Could you check a few things on this model? Use its own coordinates, in mm. A direction names the side the tool comes from. Give positions to 0.01 mm unless a question says otherwise; leave off trailing zeros. Order: outer loops, then holes, each group sorted by start corner. A loop starts at its lowest first (then second) coordinate and runs counter-clockwise, first axis right, second up. Notation, with made-up numbers: M -32.5,-37.75 L -20.5,-37.75 A15 ccw -20.5,-26.75 Z; hole C 78.5,-13.5 d11. An arc over 180 degrees is marked long. Use a Markdown table: item, result. Add a question column.
Item 1: I'm going to push flat-ended pins straight in: pin 1 Ø6 at (x, y) = (13, 15) entering from -Z; pin 2 Ø2.5 at (y, z) = (12.8, 17.5) entering from -X; pin 3 Ø2.5 at (x, z) = (12.5, 21) entering from +Y; pin 4 Ø1 at (y, z) = (4.5, 15) entering from +X. Where does each tip first touch, or does it pass through?
Item 2: For faces 4 (the face through (5, 13, 8)), 5 (the face through (14, 24, 21)), 6 (the face through (11.633, 15.095, 18.838)), which set-ups out of +Z, -Z, +X, -X, +Y, -Y let a thin tool reach every point of the face, with its end or its side?
Item 3: Suppose I cut it at B-B on y = 7.8. Write out the boundary of the cut face in (x, z).
Item 4: Suppose I cut it at A-A on x = 12.5. Write out the boundary of the cut face in (y, z).
Item 5: If we mould it in two halves opening along X, with no side actions, what happens to faces 1 (the face through (12, 19, 12.5)), 2 (the face through (12, 13, 25)), 3 (the face through (5, 3, 18))? For each: released by +X, released by -X, zero draft, split by the parting line, or undercut.
Item 6: If I drill on L1, parallel to Y at x = 16, z = 12.25; L2, parallel to Z at x = 15.5, y = 7.8; L3, parallel to X at y = 24.3, z = 21, over which ranges is the centre line in solid material (lowest first)? Write a range as from..to.
Item 7: Suppose I cut it at D-D on x = 4.5. Write out the boundary of the cut face in (y, z).
Item 8: Suppose I cut it at C-C on z = 11.5. Write out the boundary of the cut face in (x, y), plus the area to 4 significant figures.
from build123d import *

# Parameters (mm, degrees)
F0_W     = 25
F0_H     = 25
F1_DEPTH = 25
F2_R     = 4
F3_DEPTH = 12.5
F4_R     = 1.5
F5_DEPTH = 6
F6_R     = 1.5
F7_DEPTH = 5
F8_R     = 5.05
F9_DEPTH = 25.001


with BuildPart() as f1:
    # F0 (on Top) → F1 (new body)
    with BuildSketch(Plane.XY):
        with Locations((12.5, 12.5)):
            Rectangle(F0_W, F0_H)
    extrude(amount=F1_DEPTH)

    # F2 (on face) → F3 (cut)
    with BuildSketch(Plane.XY.offset(25)):
        with Locations((12.5, 19)):
            Circle(F2_R)
    extrude(amount=-F3_DEPTH, mode=Mode.SUBTRACT)

    # F4 (on face) → F5 (cut)
    with BuildSketch(Plane(origin=(0, 25, 0), x_dir=(-1, 0, 0), z_dir=(0, 1, 0))):
        with Locations((-12.5, 21)):
            Circle(F4_R)
    extrude(amount=-F5_DEPTH, mode=Mode.SUBTRACT)

    # F6 (on face) → F7 (cut)
    with BuildSketch(Plane(origin=(0, 0, 0), x_dir=(0, -1, 0), z_dir=(-1, 0, 0))):
        with Locations((-2.8, 7.5)):
            Circle(F6_R)
        with Locations((-2.8, 17.5)):
            Circle(F6_R)
        with Locations((-12.8, 7.5)):
            Circle(F6_R)
        with Locations((-12.8, 17.5)):
            Circle(F6_R)
    extrude(amount=-F7_DEPTH, mode=Mode.SUBTRACT)

    # F8 (on face) → F9 (cut, through all)
    with BuildSketch(Plane(origin=(0, 0, 0), x_dir=(0, -1, 0), z_dir=(-1, 0, 0))):
        with Locations((-7.8, 12.5)):
            Circle(F8_R)
    extrude(amount=-F9_DEPTH, mode=Mode.SUBTRACT)


solid = f1.part
Findings below:
| question | item | result |
|---|---|---|
| 1 | pin 1 | stops at z = 0 |
| 1 | pin 2 | stops at x = 5 |
| 1 | pin 3 | stops at y = 15.2 |
| 1 | pin 4 | passes through |
| 2 | face 4 | -X |
| 2 | face 5 | +Y |
| 2 | face 6 | +Z |
| 3 | outline | M 0,0 L 25,0 L 25,7.45 L 0,7.45 Z; M 0,17.55 L 25,17.55 L 25,25 L 0,25 Z |
| 4 | outline | M 0,0 L 25,0 L 25,19.5 L 23,19.5 L 23,12.5 L 15,12.5 L 15,25 L 0,25 Z; M 23,22.5 L 25,22.5 L 25,25 L 23,25 Z; hole C 7.8,12.5 d10.1 |
| 5 | face 1 | undercut |
| 5 | face 2 | zero draft |
| 5 | face 3 | released by -X |
| 6 | L1 | y = 0..2.76, 12.84..25 |
| 6 | L2 | z = 0..7.45, 17.55..25 |
| 6 | L3 | x = 0..11, 14..25 |
| 7 | outline | M 0,0 L 25,0 L 25,25 L 0,25 Z; hole C 2.8,7.5 d3; hole C 2.8,17.5 d3; hole C 7.8,12.5 d10.1; hole C 12.8,7.5 d3; hole C 12.8,17.5 d3 |
| 8 | outline | M 0,0 L 25,0 L 25,2.85 L 0,2.85 Z; M 0,12.75 L 25,12.75 L 25,25 L 0,25 Z |
| 8 | area | 377.5 mm^2 |
